For this review, take the finished solid that the model builds, in its own axes (mm). A direction names the side the tool comes from. Coordinates: 2 decimals unless noted, no trailing zeros. Loops run counter-clockwise (first coordinate to the right, second up) from the corner with the lowest first, then second, coordinate; pieces in that order, holes last. Notation, with made-up numbers: (51.25, 11.5) - (87.25, 11.5) arc R28 cw to (87.25, 30.5) - close; hole circle Ø3 at (26.5, 3.25). An arc over 180 degrees is marked (long way). Use one line per item in the form item = value. Start each with the question number.
1. Add section C-C on y = 2. Give the boundary of the cut face in (x, z), and give its area (3 significant figures).
2. Add section B-B on z = 0. Give the boundary of the cut face in (x, y), and give its area (3 significant figures).
3. Add section A-A on x = 13.5. Give the boundary of the cut face in (y, z).
4. Add section D-D on z = -3. Give the boundary of the cut face in (x, y).
5. Draft analysis for pull direction X (two halves, no side actions). For faces 1 (the face through (0, 1, -2)), 2 (the face through (-17.5, 5, 0)), 3 (the face through (0, 0, -3)), state which applies: +X half, -X half, draft (parallel to the pull), parting line (faces both ways), or undercut.
6. To check wall thickness, follow probe 1 along Z at (x, y) = (4.5, 8); probe 2 along X at (y, z) = (6.5, 0.25); probe 3 along Z at (x, y) = (9, 0.5). State the ranges of each line that lie inside material, in increasing order.
7. For pin 1 Ø6 at (x, z) = (1, 3.5) entering from +Y, flat-tipped, find the tip position at first contact; note if it passes through.
8. Machinability: for faces 4 (the face through (11.5, 6, 0)), 5 (the face through (10, 1, 0)), 6 (the face through (17.5, 5, 0)), which of the approach directions +Z, -Z, +X, -X, +Y, -Y give a long, thin tool a straight path to every point of the face, cutting with its end or side? Answer none if there is none.
```python
from build123d import *

# Parameters (mm, degrees)
SKETCH_1_W      = 35
SKETCH_1_H      = 15
SKETCH_1_R      = 1.5
SKETCH_1_W_2    = 23
SKETCH_1_H_2    = 10
EXTRUDE_1_DEPTH = 10
SKETCH_1_3_W    = 23
SKETCH_1_3_H    = 10
SKETCH_1_3_W_2  = 20
SKETCH_1_3_H_2  = 4
EXTRUDE_2_DEPTH = 3


with BuildPart() as part:
    # Sketch 1 → Extrude 1 (new body)
    with BuildSketch(Plane(origin=(0, 0, 0), x_dir=(1, 0, 0), z_dir=(0, 1, 0))):
        Rectangle(SKETCH_1_W, SKETCH_1_H)
        with Locations(Location((-13.5, 0, 0), (0, 0, 270))):
            Circle(SKETCH_1_R, mode=Mode.SUBTRACT)
        with Locations(Location((13.5, 0, 0), (0, 0, 270))):
            Circle(SKETCH_1_R, mode=Mode.SUBTRACT)
        Rectangle(SKETCH_1_W_2, SKETCH_1_H_2, mode=Mode.SUBTRACT)
    extrude(amount=EXTRUDE_1_DEPTH)

    # Sketch 1_3 → Extrude 2 (add)
    with BuildSketch(Plane(origin=(0, 0, 0), x_dir=(1, 0, 0), z_dir=(0, 1, 0))):
        Rectangle(SKETCH_1_3_W, SKETCH_1_3_H)
        Rectangle(SKETCH_1_3_W_2, SKETCH_1_3_H_2, mode=Mode.SUBTRACT)
    extrude(amount=EXTRUDE_2_DEPTH)


solid = part.part
```
Conclusion:
q1.outline = (-17.5, -7.5) - (17.5, -7.5) - (17.5, 7.5) - (-17.5, 7.5) - close; hole circle Ø3 at (-13.5, 0); hole (-10, -2) - (10, -2) - (10, 2) - (-10, 2) - close; hole circle Ø3 at (13.5, 0)
q1.area = 431 mm^2
q2.outline = (-17.5, 0) - (-15, 0) - (-15, 10) - (-17.5, 10) - close; (-12, 0) - (-10, 0) - (-10, 3) - (-11.5, 3) - (-11.5, 10) - (-12, 10) - close; (10, 0) - (12, 0) - (12, 10) - (11.5, 10) - (11.5, 3) - (10, 3) - close; (15, 0) - (17.5, 0) - (17.5, 10) - (15, 10) - close
q2.area = 69.0 mm^2
q3.outline = (0, -7.5) - (10, -7.5) - (10, -1.5) - (0, -1.5) - close; (0, 1.5) - (10, 1.5) - (10, 7.5) - (0, 7.5) - close
q4.outline = (-17.5, 0) - (17.5, 0) - (17.5, 10) - (11.5, 10) - (11.5, 3) - (-11.5, 3) - (-11.5, 10) - (-17.5, 10) - close
q5.face_1 = undercut
q5.face_2 = -X half
q5.face_3 = draft
q6.probe_1 = -7.5 to -5, 5 to 7.5
q6.probe_2 = -17.5 to -14.98, -12.02 to -11.5, 11.5 to 12.02, 14.98 to 17.5
q6.probe_3 = -7.5 to -2, 2 to 7.5
q7.pin_1 = 10
q8.face_4 = +Y
q8.face_5 = +Y, -Y
q8.face_6 = +Z, -Z, +X, +Y, -Y
